The listing builds one solid part. Answer for the finished solid, in the listing's coordinates (mm). A direction names the side the tool comes from. Coordinates: 2 decimals unless noted, no trailing zeros. Loops run counter-clockwise (first coordinate to the right, second up) from the corner with the lowest first, then second, coordinate; pieces in that order, holes last. Notation, with made-up numbers: (48, 35) - (100, 35) arc R9 cw to (100, 42) - close; hole circle Ø4 at (44.5, 40). An arc over 180 degrees is marked (long way). Return JSON: item names as keys, results as strings. Group by question number.
1. Section A-A (z = 43.5) is taken. Write down the section's boundary in (x, y).
2. Section B-B (y = 67.5) is taken. Write down the section's boundary in (x, z), and give its area (3 significant figures).
3. Which of the six approach directions +Z, -Z, +X, -X, +Y, -Y give full straight-line access (tool end or side, diameter ignored) to faces 1 (the face through (-45, 17, 10)), 2 (the face through (25.81, 21.34, 0.99)), 3 (the face through (30.944, 26.166, 8.451))?
4. Find the intervals of material crossed by line 1 along Y through (x, z) = (-42, 1.05); line 2 along Z through (x, y) = (-10, 18); line 3 along Z through (x, y) = (-78, 61), in increasing order.
5. The mould has two halves that part along X. Classify faces 4 (the face through (-11.15, 16.45, 25.87)), 5 (the face through (-25, 76, 33)), 6 (the face through (-17, 70, 7)), 7 (the face through (23, 13.617, 46)): pulls with the +X half, pulls with the -X half, needs draft (parallel to the pull), parting line crosses it, or undercut.
6. Section C-C (x = -10) is taken. Write down the section's boundary in (y, z), and give its area (3 significant figures).
7. Each of these flat-tipped pins is pushed along its axis until it touches: P1, Ø1.6, axis at x = -5.5, y = 12.5, coming from the +Z side; P2, Ø5, axis at x = 28.5, z = 12, coming from the -Y side; P3, Ø12, axis at x = -30.5, y = 11, coming from the +Z side; P4, Ø5, axis at x = -42, y = 61.25, coming from the -Z side. Where does it stop, or does it pass through?
8. Section D-D (y = 1) is taken. Write down the section's boundary in (x, z).
```python
from build123d import *
from build123d.topology import SkipClean

# Parameters (mm, degrees)
SKETCH_1_W               = 120
SKETCH_1_H               = 60
EXTRUDE_1_DEPTH          = 5
SKETCH_3_W               = 60
SKETCH_3_H               = 8
EXTRUDE_3_DEPTH          = 60
SKETCH_4_W               = 61.088110118
SKETCH_4_H               = 9
EXTRUDE_4_DEPTH          = 60
SKETCH_6_R               = 23.5
CUT_EXTRUDE_1_DEPTH      = 134.603892159
EXTRUDE_5_DEPTH          = 50
SKETCH_8_W               = 20.5
SKETCH_8_H               = 32.830920687
SKETCH_8_W_2             = 17.5
CUT_EXTRUDE_2_DEPTH      = 60
EXTRUDE_6_DEPTH          = 10
SKETCH_11_R              = 1.6
CUT_EXTRUDE_3_DEPTH      = 141.605734288
SKETCH_12_R              = 1.6
CUT_EXTRUDE_4_DEPTH      = 134.603892159
RIB_1_REACH              = 160.193
SKETCH_13_WALL_W         = 328.285335328
SKETCH_13_WALL_H         = 8
MIRROR_2_COPY_1_REACH    = 160.193
MIRROR_2_COPY_1_SKETCH_W = 328.285335328
MIRROR_2_COPY_1_SKETCH_H = 8
SKETCH_15_W              = 5
SKETCH_15_H              = 6.382962656
EXTRUDE_7_DEPTH          = 10
CHAMFER_2_SIZE           = 2
CHAMFER_3_SIZE           = 3
SKETCH_16_R              = 2.5
CUT_EXTRUDE_5_DEPTH      = 122.419950598
SKETCH_18_R              = 3.75
CUT_EXTRUDE_7_DEPTH      = 2


with BuildPart() as part:
    # 草图1 → 凸台-拉伸1 (new body)
    with BuildSketch(Plane.XY):
        with Locations((-25, 50)):
            Rectangle(SKETCH_1_W, SKETCH_1_H)
    extrude(amount=EXTRUDE_1_DEPTH)

    # 草图3 → 凸台-拉伸3 (add)
    with BuildSketch(Plane.XY.offset(5)):
        with Locations((5, 76)):
            Rectangle(SKETCH_3_W, SKETCH_3_H)
    extrude(amount=EXTRUDE_3_DEPTH)

    # 草图4 → 凸台-拉伸4 (add)
    with BuildSketch(Plane(origin=(35, 0, 0), x_dir=(0, 0, -1), z_dir=(1, 0, 0))):
        with Locations((-30.544055059, 18.117037344)):
            Rectangle(SKETCH_4_W, SKETCH_4_H)
    extrude(amount=-EXTRUDE_4_DEPTH)

    # 草图6 → 切除-拉伸1 (cut, through all)
    with BuildSketch(Plane(origin=(0, 0, 0), x_dir=(-1, 0, 0), z_dir=(0, 0, -1))):
        with Locations((-5, -9.213883343)):
            Circle(SKETCH_6_R)
    extrude(amount=-CUT_EXTRUDE_1_DEPTH, mode=Mode.SUBTRACT)

    # 草图7 → 凸台-拉伸5 (add)
    with SkipClean():  # the faces are left unmerged after this step: merging them gives an invalid solid
        with BuildSketch(Plane(origin=(0, 0, 0), x_dir=(-1, 0, 0), z_dir=(0, 0, -1))):
            with BuildLine():
                Line((-10.567680001, 13.617037344), (-35, 13.617037344))
                Line((-35, 13.617037344), (-35, -9.213883343))
                Line((-35, -9.213883343), (-28.586195427, -9.213883343))
                ThreePointArc((-28.586195427, -9.213883343), (-28.52007955, -8.938912115), (-28.493409427, -8.657364267))
                ThreePointArc((-28.493409427, -8.657364267), (-23.307757139, 5.51961687), (-10.567680001, 13.617037344))
            make_face()
            with BuildLine():
                Line((25, 13.617037344), (0.567680001, 13.617037344))
                ThreePointArc((0.567680001, 13.617037344), (13.307757139, 5.51961687), (18.493409427, -8.657364267))
                ThreePointArc((18.493409427, -8.657364267), (18.52007955, -8.938912115), (18.586195427, -9.213883343))
                Line((18.586195427, -9.213883343), (25, -9.213883343))
                Line((25, -9.213883343), (25, 13.617037344))
            make_face()
            with BuildLine():
                Line((25, -9.213883343), (18.586195427, -9.213883343))
                ThreePointArc((18.586195427, -9.213883343), (18.684669265, -9.464686705), (18.815961295, -9.699977643))
                Line((18.815961295, -9.699977643), (25, -19.213883343))
                Line((25, -19.213883343), (25, -9.213883343))
            make_face()
            with BuildLine():
                Line((-28.586195427, -9.213883343), (-35, -9.213883343))
                Line((-35, -9.213883343), (-35, -19.213883343))
                Line((-35, -19.213883343), (-28.815961295, -9.699977643))
                ThreePointArc((-28.815961295, -9.699977643), (-28.684669265, -9.464686705), (-28.586195427, -9.213883343))
            make_face()
        extrude(amount=-EXTRUDE_5_DEPTH)

    # 草图8 → 切除-拉伸2 (cut)
    with SkipClean():  # the faces are left unmerged after this step: merging them gives an invalid solid
        with BuildSketch(Plane(origin=(35, 0, 0), x_dir=(0, 0, -1), z_dir=(1, 0, 0))):
            with Locations((-39.75, -2.798423)):
                Rectangle(SKETCH_8_W, SKETCH_8_H)
            with Locations((-8.75, -2.798423)):
                Rectangle(SKETCH_8_W_2, SKETCH_8_H)
        extrude(amount=-CUT_EXTRUDE_2_DEPTH, mode=Mode.SUBTRACT)

    # 草图9 → 凸台-拉伸6 (add)
    with SkipClean():  # the faces are left unmerged after this step: merging them gives an invalid solid
        with BuildSketch(Plane.XZ.offset(-20)):
            with BuildLine():
                Line((-32.5, 0), (-41.5, 0))
                Line((-41.5, 0), (-44, 0))
                Line((-44, 0), (-44, 40))
                Line((-44, 40), (-41.5, 40))
                Line((-41.5, 40), (-41.5, 35.5))
                ThreePointArc((-41.5, 35.5), (-37, 31), (-32.5, 35.5))
                Line((-32.5, 35.5), (-32.5, 40))
                Line((-32.5, 40), (-30, 40))
                Line((-30, 40), (-30, 0))
                Line((-30, 0), (-32.5, 0))
            make_face()
        extrude(amount=EXTRUDE_6_DEPTH)

    # 草图11 → 切除-拉伸3 (cut, through all)
    with SkipClean():  # the faces are left unmerged after this step: merging them gives an invalid solid
        with BuildSketch(Plane(origin=(0, 72, 0), x_dir=(-1, 0, 0), z_dir=(0, -1, 0))):
            with Locations(Location((-20, -52.088110118, 0), (0, 0, 90))):
                Circle(SKETCH_11_R)
            with Locations(Location((10, -28.088110118, 0), (0, 0, 90))):
                Circle(SKETCH_11_R)
            with Locations(Location((-20, -28.088110118, 0), (0, 0, 90))):
                Circle(SKETCH_11_R)
            with Locations(Location((10, -52.088110118, 0), (0, 0, 90))):
                Circle(SKETCH_11_R)
        extrude(amount=-CUT_EXTRUDE_3_DEPTH, mode=Mode.SUBTRACT)

    # 草图12 → 切除-拉伸4 (cut, through all)
    with SkipClean():  # the faces are left unmerged after this step: merging them gives an invalid solid
        with BuildSketch(Plane(origin=(0, 0, 0), x_dir=(-1, 0, 0), z_dir=(0, 0, -1))):
            with Locations((42, 40.25)):
                Circle(SKETCH_12_R)
            with Locations((42, 61.25)):
                Circle(SKETCH_12_R)
            with Locations((72, 40.25)):
                Circle(SKETCH_12_R)
            with Locations((72, 61.25)):
                Circle(SKETCH_12_R)
        extrude(amount=-CUT_EXTRUDE_4_DEPTH, mode=Mode.SUBTRACT)

    # 草图13 wall → 筋1 (add, up to next)
    with BuildSketch(Plane(origin=(35, 68.5, 8.5), x_dir=(0, 0.707106781187, 0.707106781187), z_dir=(0, -0.707106781187, 0.707106781187)), mode=Mode.PRIVATE) as rib_1_sk1:
        with Locations((0, 4)):
            Rectangle(SKETCH_13_WALL_W, SKETCH_13_WALL_H)
    rib_1_tool1 = extrude(rib_1_sk1.sketch, amount=-RIB_1_REACH, mode=Mode.PRIVATE) - part.part
    rib_1 = rib_1_tool1.solids().sort_by_distance((35, 68.5, 8.5))[0]
    add(rib_1)

    # 镜向1: 筋1 across plane
    with SkipClean():  # the faces are left unmerged after this step: merging them gives an invalid solid
        add(rib_1.mirror(Plane(origin=(5, 0, 0), x_dir=(0, 0, 1), z_dir=(1, 0, 0))))

    # 镜向2: 筋1 across plane
    with SkipClean():  # the faces are left unmerged after this step: merging them gives an invalid solid
        add(rib_1.mirror(Plane(origin=(0, 47.308518672, 0), x_dir=(0, 0, 1), z_dir=(0, -1, 0))))

    # 镜向2 copy 1 sketch → 镜向2 copy 1 (add, up to next)
    with BuildSketch(Plane(origin=(-25, 26.117037344, 8.5), x_dir=(0, -0.7071067811870001, 0.7071067811869999), z_dir=(0, 0.7071067811869999, 0.7071067811870001)), mode=Mode.PRIVATE) as mirror_2_copy_1_sk1:
        with Locations((0, 4)):
            Rectangle(MIRROR_2_COPY_1_SKETCH_W, MIRROR_2_COPY_1_SKETCH_H)
    mirror_2_copy_1_tool1 = extrude(mirror_2_copy_1_sk1.sketch, amount=-MIRROR_2_COPY_1_REACH, mode=Mode.PRIVATE) - part.part
    add(mirror_2_copy_1_tool1.solids().sort_by_distance((-25, 26.117037344, 8.5))[0])

    # 草图15 → 凸台-拉伸7 (add)
    with SkipClean():  # the faces are left unmerged after this step: merging them gives an invalid solid
        with BuildSketch(Plane(origin=(0, 0, 0), x_dir=(-1, 0, 0), z_dir=(0, 0, -1))):
            with Locations((27.5, 16.808518672)):
                Rectangle(SKETCH_15_W, SKETCH_15_H)
            with Locations((46.5, 16.808518672)):
                Rectangle(SKETCH_15_W, SKETCH_15_H)
        extrude(amount=-EXTRUDE_7_DEPTH)

    # 倒角2
    chamfer_2_edges = [part.edges().sort_by_distance(p)[0] for p in [
        (-49, 16.808518672, 10),
    ]]
    chamfer(chamfer_2_edges, length=CHAMFER_2_SIZE)

    # 倒角3
    chamfer_3_edges = [part.edges().sort_by_distance(p)[0] for p in [
        (-25, 76, 65),
        (35, 76, 65),
        (35, 18.117037344, 61.088110118),
        (-25, 18.117037344, 61.088110118),
    ]]
    chamfer(chamfer_3_edges, length=CHAMFER_3_SIZE)

    # 草图16 → 切除-拉伸5 (cut, through all)
    with SkipClean():  # the faces are left unmerged after this step: merging them gives an invalid solid
        with BuildSketch(Plane(origin=(0, 22.617037344, 0), x_dir=(1, 0, 0), z_dir=(0, 1, 0))):
            with Locations(Location((20, -52.088110118, 0), (0, 0, 180))):
                Circle(SKETCH_16_R)
            with Locations(Location((-10, -52.088110118, 0), (0, 0, 180))):
                Circle(SKETCH_16_R)
            with Locations(Location((-10, -28.088110118, 0), (0, 0, 180))):
                Circle(SKETCH_16_R)
            with Locations(Location((20, -28.088110118, 0), (0, 0, 180))):
                Circle(SKETCH_16_R)
        extrude(amount=-CUT_EXTRUDE_5_DEPTH, mode=Mode.SUBTRACT)

    # 草图18 → 切除-拉伸7 (cut)
    with SkipClean():  # the faces are left unmerged after this step: merging them gives an invalid solid
        with BuildSketch(Plane(origin=(0, 0, 0), x_dir=(-1, 0, 0), z_dir=(0, 0, -1))):
            with Locations((75, 75)):
                Circle(SKETCH_18_R)
            with Locations((25, 75)):
                Circle(SKETCH_18_R)
            with Locations((-25, 75)):
                Circle(SKETCH_18_R)
            with Locations((-25, 25)):
                Circle(SKETCH_18_R)
            with Locations((25, 25)):
                Circle(SKETCH_18_R)
            with Locations((75, 25)):
                Circle(SKETCH_18_R)
        extrude(amount=-CUT_EXTRUDE_7_DEPTH, mode=Mode.SUBTRACT)


solid = part.part
```
The answers:
{
 "1": {"outline": "(-25, 13.62) - (-0.57, 13.62) arc R23.5 cw to (10.57, 13.62) - (35, 13.62) - (35, 22.62) - (-25, 22.62) - close; (-25, 72) - (35, 72) - (35, 80) - (-25, 80) - close"},
 "2": {"outline": "(-85, 0) - (35, 0) - (35, 7.5) - (27, 7.5) - (27, 5) - (-17, 5) - (-17, 7.5) - (-25, 7.5) - (-25, 5) - (-85, 5) - close", "area": "640 mm2"},
 "3": {"face 1": "+Z, -X, +Y, -Y", "face 2": "-Z", "face 3": "+Z, +X, -X"},
 "4": {"line 1": "y = 10 to 38.65, 41.85 to 59.65, 62.85 to 80", "line 2": "z = 0 to 25.59, 30.59 to 49.59, 54.59 to 61.09", "line 3": "z = 0 to 5"},
 "5": {"face 4": "undercut", "face 5": "pulls with the -X half", "face 6": "undercut", "face 7": "needs draft"},
 "6": {"outline": "(8.88, 17.5) - (13.62, 17.5) - (13.62, 0) - (80, 0) - (80, 26.49) - (72, 26.49) - (72, 5) - (22.62, 5) - (22.62, 25.59) - (8.88, 25.59) - close; (13.62, 30.59) - (22.62, 30.59) - (22.62, 49.59) - (13.62, 49.59) - close; (13.62, 54.59) - (22.62, 54.59) - (22.62, 61.09) - (13.62, 61.09) - close; (72, 29.69) - (80, 29.69) - (80, 50.49) - (72, 50.49) - close; (72, 53.69) - (80, 53.69) - (80, 65) - (72, 65) - close", "area": "1,210 mm2"},
 "7": {"P1": "stops at z = 29.5", "P2": "stops at y = 13.62", "P3": "stops at z = 40", "P4": "stops at z = 0"},
 "8": {"outline": "(-25, 17.5) - (-16.16, 17.5) - (-16.16, 29.5) - (-25, 29.5) - close; (26.16, 17.5) - (35, 17.5) - (35, 29.5) - (26.16, 29.5) - close"}
}
